Source: CAD feature listing. Evaluate the final solid. Frame: model axes, mm. A direction names the side the tool comes from. Give positions to 0.01 mm unless a question says otherwise; leave off trailing zeros. Loops run counter-clockwise (first coordinate to the right, second up) from the corner with the lowest first, then second, coordinate; pieces in that order, holes last. Notation, with made-up numbers: (-29.5, 86) -> (4.5, 86) arc R25 ccw to (4.5, 110) -> close; hole circle Ø1 at (1, 17.5). An arc over 180 degrees is marked (long way). Return JSON: item names as keys, results as strings. Group by question number.
(1) Cut plane C-C on y = 3.75. Return loops of the section in (x, z), then the cut area to 3 significant figures.
(2) Cut plane A-A on y = 11. Return loops of the section in (x, z).
(3) Pin query (flat end, axial travel): pin 1 (17 mm diameter, centred on x = 11, z = 2, fed in from +Y); pin 2 (8 mm diameter, centred on x = 7.5, y = 13, fed in from +Z); pin 3 (1.5 mm diameter, centred on x = 0, z = -5, fed in from -Y); pin 4 (10 mm diameter, centred on y = 13.5, z = 19.5, fed in from -X). Return the tip coordinate at first contact, or that it passes through.
(4) Ray query, line 1 (Z direction, x = 0, y = 11.55); line 2 (Z direction, x = 0, y = 4.5). Return the intervals inside material, ascending. Write a range as from..to.
(5) Access query for faces 5 (the face through (5.47, 16.04, 24.65)), 6 (the face through (0, 0, 0)), 7 (the face through (2.539, 10.986, -19.334)). Directions: +Z, -Z, +X, -X, +Y, -Y. A direction counts if a zero-diameter tool reaches every point of the face in a straight line with its end or side. Return the directions, or none.
(6) Draft query along Z for faces 1 (the face through (-11, 12, 17)), 2 (the face through (0.27, 6.45, -3.78)), 3 (the face through (-15.19, 9.56, -23.82)), 4 (the face through (-19, 23.5, -9)). Return one class per face: released by +Z, released by -Z, zero draft, split by the parting line, or undercut.
(7) Cut plane B-B on z = 0. Return loops of the section in (x, y), then the cut area to 3 significant figures.
```python
from build123d import *

# Parameters (mm, degrees)
M3X0_51_D     = 2.5
M3X0_51_DEPTH = 7
M3X0_51_TIP   = 0.751075774


with BuildPart() as part:
    # Эскиз1 → Повернуть1 (revolve)
    with BuildSketch(Plane.XY):
        Polygon((0, 0), (-29.5, 0), (-30.5, 1), (-30.5, 5), (-30, 5.5), (-28.25, 5.5), (-28.25, 13.5), (-25.25, 13.5), (-25.25, 18.5), (-28.25, 18.5), (-28.25, 23.5), (-20.5, 23.5), (-20.5, 12), (-19.5, 12), (-19.5, 10), (0, 10), align=None)
    revolve(axis=Axis((0, 10, 0), (0, -1, 0)))

    # Отверстие обработанное метчиком M3x0.51
    with Locations(Plane(origin=(0, 10, -5), x_dir=(1, 0, 0), z_dir=(0, 1, 0))):
        with Locations((0, 0)):
            Hole(M3X0_51_D / 2, depth=M3X0_51_DEPTH)
            with Locations((0, 0, -(M3X0_51_DEPTH + M3X0_51_TIP / 2))):  # 118° drill point
                Cone(0, M3X0_51_D / 2, M3X0_51_TIP, mode=Mode.SUBTRACT)


solid = part.part
```
Answers:
{
 "1": {"outline": "circle Ø61 at (0, 0); hole circle Ø2.5 at (0, -5)", "area": "2,920 mm²"},
 "2": {"outline": "circle Ø56.5 at (0, 0); hole circle Ø39 at (0, 0)"},
 "3": {"pin 1": "y = 12", "pin 2": "z = 28.03", "pin 3": "y = 0", "pin 4": "x = -24.24"},
 "4": {"line 1": "-28.25..-19.5, 19.5..28.25", "line 2": "-30.5..-6.25, -3.75..30.5"},
 "5": {"face 5": "none", "face 6": "+Z, -Z, +X, -X, -Y", "face 7": "+Y"},
 "6": {"face 1": "undercut", "face 2": "undercut", "face 3": "split by the parting line", "face 4": "zero draft"},
 "7": {"outline": "(-30.5, 1) -> (-29.5, 0) -> (29.5, 0) -> (30.5, 1) -> (30.5, 5) -> (30, 5.5) -> (28.25, 5.5) -> (28.25, 13.5) -> (25.25, 13.5) -> (25.25, 18.5) -> (28.25, 18.5) -> (28.25, 23.5) -> (20.5, 23.5) -> (20.5, 12) -> (19.5, 12) -> (19.5, 10) -> (-19.5, 10) -> (-19.5, 12) -> (-20.5, 12) -> (-20.5, 23.5) -> (-28.25, 23.5) -> (-28.25, 18.5) -> (-25.25, 18.5) -> (-25.25, 13.5) -> (-28.25, 13.5) -> (-28.25, 5.5) -> (-30, 5.5) -> (-30.5, 5) -> close", "area": "772 mm²"}
}
